For this review, take the finished solid that the model builds, in its own axes (mm). A direction names the side the tool comes from. Round coordinates to 2 decimals unless told otherwise and drop trailing zeros. Write each loop counter-clockwise with the first axis right and the second up, starting at its lowest first coordinate (ties: lowest second). Pieces come first, ordered by that corner, then holes. Notation, with made-up numbers: (33, 75.25) -> (70, 75.25) arc R22 cw to (70, 94.25) -> close; hole circle Ø6 at (88.5, -34). An arc over 180 degrees is marked (long way). Answer in a Markdown table with one row per item.
from build123d import *

# Parameters (mm, degrees)
F1_DEPTH = 6
F3_DEPTH = 10
F4_W     = 20
F4_H     = 6
F5_DEPTH = 10
F7_DEPTH = 25
F8_DEPTH = 4


with BuildPart() as f1:
    # F0 (on Top) → F1 (new body)
    with BuildSketch(Plane.XY):
        Polygon((0, -20), (0, 0), (-20, 0), align=None)
    extrude(amount=F1_DEPTH)

    # F3 (add): a face of the model
    f3_faces = [f1.faces().sort_by_distance(p)[0] for p in [
        (-10, 0, 3),
    ]]
    extrude(f3_faces, amount=F3_DEPTH)

    # F4 (on face) → F5 (join)
    with BuildSketch(Plane.YZ):
        with Locations((-10, 3)):
            Rectangle(F4_W, F4_H)
    extrude(amount=F5_DEPTH)

    # F6 (on face) → F7 (cut)
    with BuildSketch(Plane.XY.offset(6)):
        with BuildLine():
            ThreePointArc((-2, -5), (-6.1480502971, -2.2283614025), (-7.1213203436, -7.1213203436))
            ThreePointArc((-7.1213203436, -7.1213203436), (-3.8519497029, -7.7716385975), (-2, -5))
        make_face()
    extrude(amount=-F7_DEPTH, mode=Mode.SUBTRACT)

    # F6 (on face) → F8 (join)
    with BuildSketch(Plane.XY.offset(6)):
        Polygon((-20, 0), (-10, -10), (0, -20), (10, -20), (10, 0), (0, 0), (0, 10), (-20, 10), align=None)
        with BuildLine():
            ThreePointArc((0.75, -5), (-2.7995702639, -10.3123073119), (-9.0658639918, -9.0658639918))
            ThreePointArc((-9.0658639918, -9.0658639918), (-7.2004297361, 0.3123073119), (0.75, -5))
        make_face(mode=Mode.SUBTRACT)
    extrude(amount=F8_DEPTH)


solid = f1.part
1) Consider section C-C on z = 7.75. State the section outline as (x, y) points, then the cut area to 3 significant figures.
Solved:
| item | result |
|---|---|
| outline | (-20, 0) -> (0, -20) -> (10, -20) -> (10, 0) -> (0, 0) -> (0, 10) -> (-20, 10) -> close; hole circle Ø11.5 at (-5, -5) |
| area | 496 mm² |
2) Mouldability with a two-part tool opening along Y and no side actions: class faces 1 (the flat face through (-2.5, -2.5, 6)), 2 (the flat face through (10, -10, 5)), 3 (the flat face through (-10, 10, 5)) as pulls with the +Y half, pulls with the -Y half, needs draft (parallel to the pull), parting line crosses it, or undercut.
Solved:
| item | result |
|---|---|
| face 1 | undercut |
| face 2 | needs draft |
| face 3 | pulls with the +Y half |
3) Consider section D-D on y = -17.5. State the section outline as (x, z) points.
Solved:
| item | result |
|---|---|
| outline | (-2.5, 0) -> (10, 0) -> (10, 10) -> (-2.5, 10) -> close |
4) Consider section A-A on x = -5. State the section outline as (y, z) points.
Solved:
| item | result |
|---|---|
| outline | (-15, 0) -> (-8, 0) -> (-8, 6) -> (-10.75, 6) -> (-10.75, 10) -> (-15, 10) -> close; (-2, 0) -> (10, 0) -> (10, 10) -> (0.75, 10) -> (0.75, 6) -> (-2, 6) -> close |
5) For faces 4 (the flat face through (0, 5, 5)), 5 (the flat face through (1, -1, 10)), list the 3-axis set-ups (+Z, -Z, +X, -X, +Y, -Y) from which the entire face can be reached by the end or side of a thin tool; tool diameter is ignored.
Solved:
| item | result |
|---|---|
| face 4 | +Z, -Z, +X, +Y |
| face 5 | +Z, +X, -X, +Y, -Y |
6) Consider section B-B on z = 5.25. State the section outline as (x, y) points.
Solved:
| item | result |
|---|---|
| outline | (-20, 0) -> (0, -20) -> (10, -20) -> (10, 0) -> (0, 0) -> (0, 10) -> (-20, 10) -> close; hole circle Ø6 at (-5, -5) |
7) For line 1 (X direction, y = 4, z = 3); line 2 (X direction, y = -7.5, z = 8); line 3 (Y direction, x = -5, z = 8.75), list the stretches that pass through material, from the lowest coordinate up. Write a range as [from, to].
Solved:
| item | result |
|---|---|
| line 1 | [-20, 0] |
| line 2 | [-12.5, -10.18], [0.18, 10] |
| line 3 | [-15, -10.75], [0.75, 10] |
8) Clearance check with flat-ended pins moving along their axes: pin 1 Ø10 at (x, y) = (-2.5, 0) entering from -Z; pin 2 Ø5 at (x, y) = (-5, -5) entering from -Z; pin 3 Ø5 at (y, z) = (-3, 5) entering from -X; pin 4 Ø1 at (x, z) = (-8, 4.5) entering from -Y. State where each tip first meets the part, or that it passes through.
Solved:
| item | result |
|---|---|
| pin 1 | z = 0 |
| pin 2 | through |
| pin 3 | x = -19.5 |
| pin 4 | y = -12.5 |
